Part model, mm, in its own coordinate system. Face numbers are marked on the shaded views. A direction names the side the tool comes from. Give positions to 0.01 mm unless a question says otherwise; leave off trailing zeros. Loops run counter-clockwise (first coordinate to the right, second up) from the corner with the lowest first, then second, coordinate; pieces in that order, holes last. Notation, with made-up numbers: M 27,70.5 L 53,70.5 A21 cw 53,88.5 Z; hole C 50.5,36 d8. An arc over 180 degrees is marked long. Put each result on its own line as item: value. Start each with the question number.
```python
from build123d import *

# Parameters (mm, degrees)
SKETCH_1_R          = 9.5
EXTRUDE_1_DEPTH     = 5
SKETCH_2_R          = 8
EXTRUDE_2_DEPTH     = 11.5
EXTRUDE_3_DEPTH     = 3
SKETCH_4_R          = 9.5
EXTRUDE_4_DEPTH     = 3
SKETCH_5_R          = 8.5
SKETCH_5_R_2        = 1
CUT_EXTRUDE_2_DEPTH = 6


with BuildPart() as part:
    # 草图1 → 凸台-拉伸1 (new body)
    with BuildSketch(Plane.XY):
        Circle(SKETCH_1_R)
    extrude(amount=EXTRUDE_1_DEPTH)

    # 草图2 → 凸台-拉伸2 (add)
    with BuildSketch(Plane(origin=(0, 0, 0), x_dir=(-1, 0, 0), z_dir=(0, 0, -1))):
        with Locations(Location((0, 0, 0), (0, 0, 180))):
            Circle(SKETCH_2_R)
    extrude(amount=EXTRUDE_2_DEPTH)

    # 草图3 → 凸台-拉伸3 (add)
    with BuildSketch(Plane(origin=(0, 0, 0), x_dir=(-1, 0, 0), z_dir=(0, 0, -1))):
        Polygon((0, 10.969655115), (-9.5, 5.484827557), (-9.5, -5.484827557), (0, -10.969655115), (9.5, -5.484827557), (9.5, 5.484827557), align=None)
    extrude(amount=-EXTRUDE_3_DEPTH)

    # 草图4 → 凸台-拉伸4 (add)
    with BuildSketch(Plane.XY.offset(5)):
        Circle(SKETCH_4_R)
    extrude(amount=EXTRUDE_4_DEPTH)

    # 草图5 → 切除-拉伸2 (cut)
    with BuildSketch(Plane.XY.offset(8)):
        Circle(SKETCH_5_R)
        with Locations((2.598076211, 1.5)):
            Circle(SKETCH_5_R_2, mode=Mode.SUBTRACT)
        with Locations((-2.598076211, -1.5)):
            Circle(SKETCH_5_R_2, mode=Mode.SUBTRACT)
    extrude(amount=-CUT_EXTRUDE_2_DEPTH, mode=Mode.SUBTRACT)


solid = part.part
```
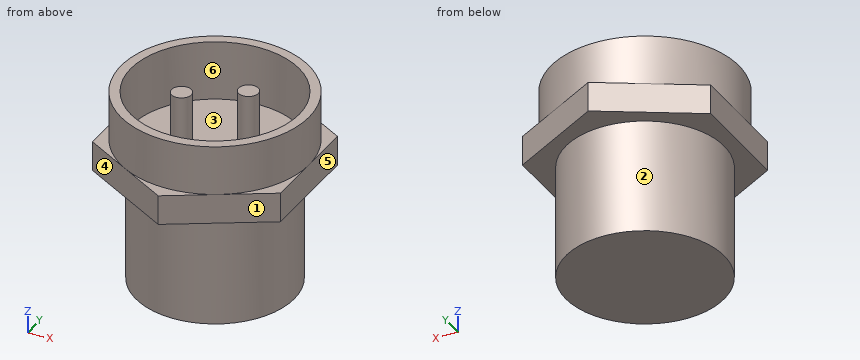
1) Which spindle directions (+Z, -Z, +X, -X, +Y, -Y) get a long thin tool onto all of the face, cutting with end or side? Do the marked faces 1, 2 and 3. Say none if no direction does.
2) Band-saw the part on B-B on z = -3.25. Give the cut face in (x, y), then the cut area to 3 significant figures.
3) Band-saw the part on D-D on y = 1.5. Give the cut face in (x, z), then the cut area to 3 significant figures.
4) Pin check, flat tips, straight feed: pin 1 Ø4 at (y, z) = (-6, -9) entering from +X; pin 2 Ø4 at (x, z) = (4, -0.5) entering from +Y. Stop position of each tip, or through.
5) Mould opens along X. For the marked faces 4, 5 and 6 say: +X half, -X half, draft (parallel to the pull), parting line (faces both ways), or undercut.
6) Wall check: L1, parallel to Y at x = 0, z = 5.5; L2, parallel to Z at x = 4.25, y = 7.75; L3, parallel to Y at x = 2, z = 2.5. Give the ranges that are in metal, low to high.
7) Band-saw the part on A-A on y = -4. Give the cut face in (x, z), then the cut area to 3 significant figures.
8) Band-saw the part on C-C on x = 1.25. Give the cut face in (y, z), then the cut area to 3 significant figures.
Evaluation:
1. face 1: +Z, -Z, +X, -Y
1. face 2: -Z
1. face 3: +Z
2. outline: C 0,0 d16
2. area: 201 mm2
3. outline: M -9.5,0 L -7.86,0 L -7.86,-11.5 L 7.86,-11.5 L 7.86,0 L 9.5,0 L 9.5,3 L 9.38,3 L 9.38,8 L 8.37,8 L 8.37,2 L 3.6,2 L 3.6,8 L 1.6,8 L 1.6,2 L -8.37,2 L -8.37,8 L -9.38,8 L -9.38,3 L -9.5,3 Z
3. area: 243 mm2
4. pin 1: x = 6.93
4. pin 2: y = 9.78
5. face 4: -X half
5. face 5: +X half
5. face 6: undercut
6. L1: -9.5 to -8.5, 8.5 to 9.5
6. L2: 0 to 8
6. L3: -9.81 to -8.26, 0.7 to 2.3, 8.26 to 9.81
7. outline: M -9.5,0 L -6.93,0 L -6.93,-11.5 L 6.93,-11.5 L 6.93,0 L 9.5,0 L 9.5,3 L 8.62,3 L 8.62,8 L 7.5,8 L 7.5,2 L -7.5,2 L -7.5,8 L -8.62,8 L -8.62,3 L -9.5,3 Z
7. area: 213 mm2
8. outline: M -10.25,0 L -7.9,0 L -7.9,-11.5 L 7.9,-11.5 L 7.9,0 L 10.25,0 L 10.25,3 L 9.42,3 L 9.42,8 L 8.41,8 L 8.41,2 L -8.41,2 L -8.41,8 L -9.42,8 L -9.42,3 L -10.25,3 Z
8. area: 237 mm2
